Check sheet for the modelled part. Datum: model origin and axes. Units: mm. A direction names the side the tool comes from. Coordinates: 2 decimals unless noted, no trailing zeros. Loops run counter-clockwise (first coordinate to the right, second up) from the corner with the lowest first, then second, coordinate; pieces in that order, holes last.
```python
from build123d import *

# Parameters (mm, degrees)
BOSS_EXTRUDE1_DEPTH      = 10
BOSS_EXTRUDE1_DEPTH_BACK = 150
SKETCH1_R                = 10
SKETCH2_R                = 30
BOSS_EXTRUDE2_DEPTH      = 10
SHELL1_START             = -149
SHELL1_OUTLINE_R         = 9
SHELL1_DEPTH             = 168
SHELL1_START_2           = 11
SHELL1_2_OUTLINE_R       = 29
SHELL1_2_OUTLINE_R_2     = 9
SHELL1_2_DEPTH           = 8


# Read off the part's stored shape, not the designer's step: Shell1
with BuildPart() as part:
    # Sketch1 → Boss-Extrude1 (new, two sides: drawn at the far end of the back side and taken through both)
    with BuildSketch(Plane.XY.offset(-BOSS_EXTRUDE1_DEPTH_BACK)):
        Circle(SKETCH1_R)
    extrude(amount=BOSS_EXTRUDE1_DEPTH + BOSS_EXTRUDE1_DEPTH_BACK)

    # Sketch2 → Boss-Extrude2 (add)
    with BuildSketch(Plane.XY.offset(10)):
        Circle(SKETCH2_R)
    extrude(amount=BOSS_EXTRUDE2_DEPTH)

    # Shell1 outline → Shell1 (cut)
    with BuildSketch(Plane.XY.offset(SHELL1_START)):
        Circle(SHELL1_OUTLINE_R)
    extrude(amount=SHELL1_DEPTH, mode=Mode.SUBTRACT)

    # Shell1 2 outline → Shell1 2 (cut)
    with BuildSketch(Plane.XY.offset(SHELL1_START_2)):
        Circle(SHELL1_2_OUTLINE_R)
        Circle(SHELL1_2_OUTLINE_R_2, mode=Mode.SUBTRACT)
    extrude(amount=SHELL1_2_DEPTH, mode=Mode.SUBTRACT)


solid = part.part
```
1) Scan lines: line 1 (Z direction, x = 1, y = -19); line 2 (Z direction, x = 1.5, y = -6); line 3 (Y direction, x = 0, z = -25.5). Record each from-to range of solid material in increasing order.
Answer sheet:
line 1: z = 10 to 11, 19 to 20
line 2: z = -150 to -149, 19 to 20
line 3: y = -10 to -9, 9 to 10
2) Set-up check for faces 1 (the flat face through (13, 0, 10)), 2 (the flat face through (0, 0, -149)), 3 (the flat face through (0, 0, 20)): record each of +Z, -Z, +X, -X, +Y, -Y from which the full face is reachable in a straight line by a thin tool's end or side.
Answer sheet:
face 1: -Z
face 2: none
face 3: +Z, +X, -X, +Y, -Y
3) Section check C-C on z = -66. Enter the section's corners in (x, y), plus the area to 3 significant figures.
Answer sheet:
outline: circle Ø20 at (0, 0); hole circle Ø18 at (0, 0)
area: 59.7 mm2
4) Depth check by flat-ended pin: pin 1 (12 mm diameter, centred on x = 3.5, z = -46, fed in from -Y); pin 2 (1.5 mm diameter, centred on y = -1, z = -76.5, fed in from -X); pin 3 (5 mm diameter, centred on y = 3, z = -96.5, fed in from +X). Enter the tip coordinate at first touch or a pass-through.
Answer sheet:
pin 1: stops at y = -10
pin 2: stops at x = -10
pin 3: stops at x = 9.99
5) Section check A-A on y = 0. Enter the section's corners in (x, z).
Answer sheet:
outline: (-30, 10) - (-10, 10) - (-10, -150) - (10, -150) - (10, 10) - (30, 10) - (30, 20) - (-30, 20) - close; hole (-29, 11) - (-9, 11) - (-9, -149) - (9, -149) - (9, 11) - (29, 11) - (29, 19) - (-29, 19) - close
6) Section check D-D on x = 17. Enter the section's corners in (y, z), plus the area to 3 significant figures.
Answer sheet:
outline: (-24.72, 10) - (24.72, 10) - (24.72, 20) - (-24.72, 20) - close; hole (-23.49, 11) - (23.49, 11) - (23.49, 19) - (-23.49, 19) - close
area: 118 mm2
7) Mould release check, pull along Y, two halves, no side actions. Record for faces 4 (the flat face through (0, 0, -150)), 5 (the cylindrical face through (-2.17, -9.76, -71.12)), 6 (the flat face through (6, 7, 11)): +Y half, -Y half, draft (parallel to the pull), parting line (faces both ways), or undercut.
Answer sheet:
face 4: draft
face 5: parting line
face 6: undercut
